Read the model definition and answer for the solid it produces. Units are mm, in the model's axes. A direction names the side the tool comes from. Coordinates: 2 decimals unless noted, no trailing zeros. Write each loop counter-clockwise with the first axis right and the second up, starting at its lowest first coordinate (ties: lowest second). Pieces come first, ordered by that corner, then holes. Notation, with made-up numbers: (53, 46) - (90, 46) arc R10 cw to (90, 56) - close; hole circle Ø10 at (-15.5, 40). An arc over 180 degrees is marked (long way). Use a Markdown table: item, result.
from build123d import *

# Parameters (mm, degrees)
SKETCH1_W           = 75
SKETCH1_H           = 40
BOSS_EXTRUDE1_DEPTH = 25
SKETCH5_W           = 56.924134656
SKETCH5_H           = 49.860042304
CUT_EXTRUDE1_DEPTH  = 19.463723647
SKETCH9_W           = 66.205259198
SKETCH9_H           = 57.927204101
CUT_EXTRUDE4_DEPTH  = 19.463723647
CUT_EXTRUDE5_DEPTH  = 10
CUT_EXTRUDE6_DEPTH  = 10
SKETCH12_R          = 5
CUT_EXTRUDE7_DEPTH  = 26
SKETCH13_R          = 5
CUT_EXTRUDE8_DEPTH  = 26
SKETCH14_W          = 20
SKETCH14_H          = 10
CUT_EXTRUDE9_DEPTH  = 26


with BuildPart() as part:
    # Sketch1 → Boss-Extrude1 (new body)
    with BuildSketch(Plane(origin=(0, 0, 0), x_dir=(1, 0, 0), z_dir=(0, 1, 0))):
        with Locations((37.5, 20)):
            Rectangle(SKETCH1_W, SKETCH1_H)
    extrude(amount=BOSS_EXTRUDE1_DEPTH)

    # Sketch5 → Cut-Extrude1 (cut, through all)
    with BuildSketch(Plane(origin=(24.621212121, 19.696969697, 24.621212121), x_dir=(-0.48059153, -0.384473224, 0.788170109), z_dir=(-0.615457455, -0.492365964, -0.615457455))):
        with Locations((-56.377268539, -29.25842023)):
            Rectangle(SKETCH5_W, SKETCH5_H)
    extrude(amount=-CUT_EXTRUDE1_DEPTH, mode=Mode.SUBTRACT)

    # Sketch9 → Cut-Extrude4 (cut, through all)
    with BuildSketch(Plane(origin=(39.772727273, 31.818181818, -39.772727273), x_dir=(-0.48059153, -0.384473224, -0.788170109), z_dir=(0.615457455, 0.492365964, -0.615457455))):
        with Locations((-25.664759868, -34.253534267)):
            Rectangle(SKETCH9_W, SKETCH9_H)
    extrude(amount=CUT_EXTRUDE4_DEPTH, mode=Mode.SUBTRACT)

    # Sketch10 → Cut-Extrude5 (cut)
    with BuildSketch(Plane.ZY):
        Polygon((-10, 25), (0, 20), (0, 25), align=None)
    extrude(amount=-CUT_EXTRUDE5_DEPTH, mode=Mode.SUBTRACT)

    # Sketch11 → Cut-Extrude6 (cut)
    with BuildSketch(Plane.ZY):
        Polygon((-40, 20), (-30, 25), (-40, 25), align=None)
    extrude(amount=-CUT_EXTRUDE6_DEPTH, mode=Mode.SUBTRACT)

    # Sketch12 → Cut-Extrude7 (cut, through all)
    with BuildSketch(Plane(origin=(0, 25, 0), x_dir=(1, 0, 0), z_dir=(0, 1, 0))):
        with Locations((25, 20)):
            Circle(SKETCH12_R)
    extrude(amount=-CUT_EXTRUDE7_DEPTH, mode=Mode.SUBTRACT)

    # Sketch13 → Cut-Extrude8 (cut, through all)
    with BuildSketch(Plane(origin=(0, 25, 0), x_dir=(1, 0, 0), z_dir=(0, 1, 0))):
        with Locations((45, 20)):
            Circle(SKETCH13_R)
    extrude(amount=-CUT_EXTRUDE8_DEPTH, mode=Mode.SUBTRACT)

    # Sketch14 → Cut-Extrude9 (cut, through all)
    with BuildSketch(Plane(origin=(0, 25, 0), x_dir=(1, 0, 0), z_dir=(0, 1, 0))):
        with Locations((35, 20)):
            Rectangle(SKETCH14_W, SKETCH14_H)
    extrude(amount=-CUT_EXTRUDE9_DEPTH, mode=Mode.SUBTRACT)


solid = part.part
(1) This flat-tipped pin is pushed along its axis until it touches: P1, Ø1.5, axis at x = 53, y = 20.5, coming from the +Z side. Where does it stop, or does it pass through?
Report:
| item | result |
|---|---|
| P1 | stops at z = -3.44 |
(2) For faces 4 (the flat face through (35, 13, -25)), 5 (the flat face through (4.93, 22.535, -5.07)), 6 (the flat face through (25, 12, 0)), 7 (the flat face through (10, 23, -36)), determine the directions among +Z, -Z, +X, -X, +Y, -Y from which every point of the face is accessible in a straight line to the end or side of a thin tool.
Report:
| item | result |
|---|---|
| face 4 | +Y, -Y |
| face 5 | +Z, -X, +Y |
| face 6 | +Z, +X, -X, +Y, -Y |
| face 7 | -Z, -X, +Y |
(3) The mould has two halves that part along Z. Classify faces 1 (the flat face through (63, 15, -30)), 2 (the flat face through (25, 25, -29)), 3 (the flat face through (35, 13, -15)): pulls with the +Z half, pulls with the -Z half, needs draft (parallel to the pull), parting line crosses it, or undercut.
Report:
| item | result |
|---|---|
| face 1 | pulls with the -Z half |
| face 2 | needs draft |
| face 3 | undercut |
(4) A cutting plane is placed at C-C, the plane x = 41. Write down the section's boundary in (y, z), and give its area (3 significant figures).
Report:
| item | result |
|---|---|
| outline | (0, -40) - (25, -40) - (25, -25) - (0, -25) - close; (0, -15) - (25, -15) - (25, 0) - (0, 0) - close |
| area | 750 mm² |
(5) Straight lines are drawn through the part: L1, parallel to Z at x = 28, y = 15.5; L2, parallel to X at y = 16.75, z = -24; L3, parallel to X at y = 7.25, z = -21. For each, find the intervals that lie inside material, in ascending order.
Report:
| item | result |
|---|---|
| L1 | z = -40 to -25, -15 to 0 |
| L2 | x = 0 to 22, 48 to 67.6 |
| L3 | x = 0 to 20.1, 49.9 to 75 |
(6) A cutting plane is placed at A-A, the plane z = -17. Write down the section's boundary in (x, y), and give its area (3 significant figures).
Report:
| item | result |
|---|---|
| outline | (0, 0) - (21, 0) - (21, 25) - (0, 25) - close; (49, 0) - (75, 0) - (75, 8.75) - (62, 25) - (49, 25) - close |
| area | 1,070 mm² |
(7) A cutting plane is placed at B-B, the plane y = 17. Write down the section's boundary in (x, z).
Report:
| item | result |
|---|---|
| outline | (0, -40) - (51.4, -40) - (71.4, -20) - (51.4, 0) - (0, 0) - close; hole (25, -25) - (45, -25) arc R5 ccw to (45, -15) - (25, -15) arc R5 ccw to start |
(8) A cutting plane is placed at D-D, the plane z = -36.5. Write down the section's boundary in (x, y), and give its area (3 significant figures).
Report:
| item | result |
|---|---|
| outline | (0, 0) - (68.5, 0) - (48.5, 25) - (10, 25) - (10, 21.75) - (0, 21.75) - close |
| area | 1,430 mm² |
